```python
from build123d import *

# Parameters (mm, degrees)
F0_W      = 50
F0_H      = 94
F1_DEPTH  = 2.5
F2_W      = 2.5
F2_H      = 10
F3_DEPTH  = 3
F4_R      = 2.5
F5_DEPTH  = 25
F6_W      = 10.5
F6_H      = 16.5188284865
F7_DEPTH  = 8.5
F8_W      = 4
F8_H      = 1
F9_DEPTH  = 3
F11_DEPTH = 82.4821715135
F12_R     = 0.5
F13_R     = 1.25
F14_DEPTH = 2.25
F16_DEPTH = 2
F18_W     = 1.5
F18_H     = 3.5
F19_DEPTH = 3
F20_R     = 1
F21_DEPTH = 6


# Not quite as in the source:
# - a fillet or chamfer that OpenCascade refuses, or shapes differently, is made with other operations: its cross-section is extruded or revolved along the edge and cut away or added


with BuildPart() as f1:
    # F0 (on Right) → F1 (new body)
    with BuildSketch(Plane.YZ):
        with Locations((25, 47)):
            Rectangle(F0_W, F0_H)
    extrude(amount=F1_DEPTH)

    # F2 (on face) → F3 (join)
    with BuildSketch(Plane.XY.offset(94)):
        with Locations((1.25, 40)):
            Rectangle(F2_W, F2_H)
        with Locations((1.25, 10)):
            Rectangle(F2_W, F2_H)
    extrude(amount=F3_DEPTH)

    # F4 (on face) → F5 (cut)
    with BuildSketch(Plane.YZ.offset(2.5)):
        with Locations((25, 40)):
            Circle(F4_R)
        with Locations((25, 54)):
            Circle(F4_R)
    extrude(amount=-F5_DEPTH, mode=Mode.SUBTRACT)

    # F6 (on face) → F7 (join)
    with BuildSketch(Plane.YZ.offset(2.5)):
        with Locations((24.75, 20.2594142432)):
            Rectangle(F6_W, F6_H)
    extrude(amount=F7_DEPTH)

    # F8 (on face) → F9 (join)
    with BuildSketch(Plane.XZ.offset(-19.5)):
        with Locations((6.5, 25.0188284865)):
            Rectangle(F8_W, F8_H)
        with Locations((6.5, 20.0188284865)):
            Rectangle(F8_W, F8_H)
        with Locations((6.5, 15.0188284865)):
            Rectangle(F8_W, F8_H)
    extrude(amount=F9_DEPTH)

    # F10 (on face) → F11 (cut, through all)
    with BuildSketch(Plane(origin=(0, 0, 14.5188284865), x_dir=(1, 0, 0), z_dir=(0, 0, -1))):
        with BuildLine():
            Line((5, -17.5), (5, -19.5))
            Line((5, -19.5), (8, -19.5))
            Line((8, -19.5), (8, -17.5))
            ThreePointArc((8, -17.5), (7.8535533906, -17.1464466094), (7.5, -17))
            Line((7.5, -17), (5.5, -17))
            ThreePointArc((5.5, -17), (5.1464466094, -17.1464466094), (5, -17.5))
        make_face()
    extrude(amount=-F11_DEPTH, mode=Mode.SUBTRACT)

    # F12
    f12_edges = [f1.edges().sort_by_distance(p)[0] for p in [
        (8.5, 16.5, 15.018828),
        (8.5, 16.5, 20.018828),
        (8.5, 16.5, 25.018828),
        (4.5, 16.5, 25.018828),
        (4.5, 16.5, 20.018828),
        (4.5, 16.5, 15.018828),
    ]]
    fillet(f12_edges, radius=F12_R)

    # F13 (on face) → F14 (join)
    with BuildSketch(Plane.YZ.offset(11)):
        with Locations((22.5, 25.5188284865)):
            Circle(F13_R)
        with Locations((22.5, 15)):
            Circle(F13_R)
    extrude(amount=F14_DEPTH)

    # F15 (on face) → F16 (cut)
    with BuildSketch(Plane.YZ.offset(13.25)):
        Polygon((22.2532600164, 25.2959672362), (22.2532600164, 24.5808176696), (22.7513108402, 24.5808176696), (22.7513108402, 25.2959672362), (23.51754345, 25.2959672362), (23.51754345, 25.7301647216), (22.7513108402, 25.7301647216), (22.7513108402, 26.4325458556), (22.2532600164, 26.4325458556), (22.2532600164, 25.7301647216), (21.5636510402, 25.7301647216), (21.5636510402, 25.2959672362), align=None)
        Polygon((22.2596314482, 14.7567068819), (22.2596314482, 14.0415573154), (22.757682272, 14.0415573154), (22.757682272, 14.7567068819), (23.5239148817, 14.7567068819), (23.5239148817, 15.1909043674), (22.757682272, 15.1909043674), (22.757682272, 15.8932855014), (22.2596314482, 15.8932855014), (22.2596314482, 15.1909043674), (21.5700224719, 15.1909043674), (21.5700224719, 14.7567068819), align=None)
    extrude(amount=-F16_DEPTH, mode=Mode.SUBTRACT)

    # F17: fillet of radius 1 on 2 edges, made by hand

    # F17_s1 → F17_t2 (revolve, cut)
    with BuildSketch(Plane.XY.offset(25.5188284865)):
        with BuildLine():
            ThreePointArc((12.25, 23.75), (12.9571067812, 23.4571067812), (13.25, 22.75))
            Line((13.25, 22.75), (13.25, 23.75))
            Line((13.25, 23.75), (12.25, 23.75))
        make_face()
    revolve(axis=Axis((13.25, 22.5, 25.5188284865), (1, 0, 0)), mode=Mode.SUBTRACT)

    # F17_s3 → F17_t4 (revolve, cut)
    with BuildSketch(Plane.XY.offset(15)):
        with BuildLine():
            ThreePointArc((12.25, 23.75), (12.9571067812, 23.4571067812), (13.25, 22.75))
            Line((13.25, 22.75), (13.25, 23.75))
            Line((13.25, 23.75), (12.25, 23.75))
        make_face()
    revolve(axis=Axis((13.25, 22.5, 15), (1, 0, 0)), mode=Mode.SUBTRACT)

    # F18 (on face) → F19 (join)
    with BuildSketch(Plane(origin=(0, 30, 0), x_dir=(-1, 0, 0), z_dir=(0, 1, 0))):
        with Locations((-9.25, 25.5901701748)):
            Rectangle(F18_W, F18_H)
        with Locations((-4.75, 25.6615988507)):
            Rectangle(F18_W, F18_H)
    extrude(amount=F19_DEPTH)

    # F20 (on face) → F21 (cut)
    with BuildSketch(Plane.YZ.offset(10)):
        with Locations((31.5, 25.5901701748)):
            Circle(F20_R)
    extrude(amount=-F21_DEPTH, mode=Mode.SUBTRACT)


solid = f1.part
```
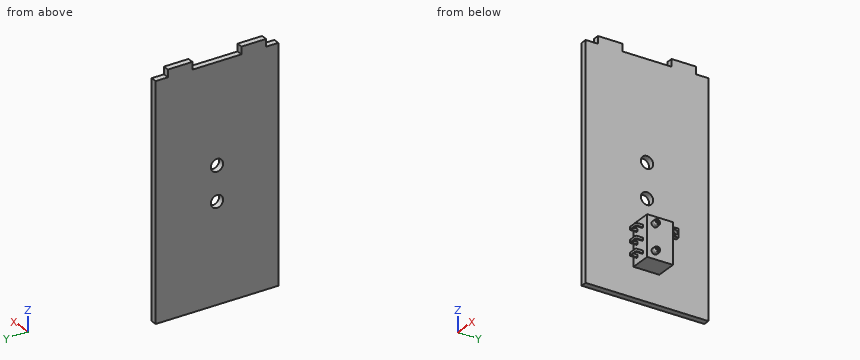
Build history of the part. All positions in model axes, mm. Give positions to 0.01 mm unless a question says otherwise; leave off trailing zeros. Order: outer loops, then holes, each group sorted by start corner. A loop starts at its lowest first (then second) coordinate and runs counter-clockwise, first axis right, second up. Notation, with made-up numbers: M -18.75,88 L -6.75,88 A18 cw -6.75,123 Z; hole C 35,17.25 d2. An arc over 180 degrees is marked long. Write item = value, one per line. Start each with the question number.
(1) Pin check, flat tips, straight feed: pin 1 Ø6 at (x, y) = (9.5, 25.5) entering from -Z; pin 2 Ø0.8 at (x, z) = (6, 15) entering from -Y; pin 3 Ø0.5 at (y, z) = (18, 15) entering from -X; pin 4 Ø0.5 at (y, z) = (18.5, 25) entering from +X. Stop position of each tip, or through.
(2) Slice it at C-C on x = 1.5. Write the cut outline in (y, z), plus the area to 3 significant figures.
(3) Slice it at A-A on y = 31.5. Write the cut outline in (x, z), plus the area to 4 significant figures.
(4) Probe L1, parallel to Z at x = 1.6, y = 25; L2, parallel to Z at x = 9.7, y = 31.5; L3, parallel to Z at x = 4.8, y = 31.5. List the from-to ranges inside material, lowest first. Write a range as [from, to].
(5) Slice it at B-B on z = 54. Write the cut outline in (x, y), plus the area to 4 significant figures.
(6) Slice it at D-D on z = 39. Write the cut outline in (x, y).
Responses:
q1.pin_1 = 12
q1.pin_2 = 16.5
q1.pin_3 = 0
q1.pin_4 = 8.5
q2.outline = M 0,0 L 50,0 L 50,94 L 45,94 L 45,97 L 35,97 L 35,94 L 15,94 L 15,97 L 5,97 L 5,94 L 0,94 Z; hole C 25,40 d5; hole C 25,54 d5
q2.area = 4,720 mm2
q3.outline = M 0,0 L 2.5,0 L 2.5,94 L 0,94 Z; M 4,23.91 L 5.5,23.91 L 5.5,24.59 L 4,24.59 Z; M 4,26.59 L 5.5,26.59 L 5.5,27.41 L 4,27.41 Z; M 8.5,23.84 L 10,23.84 L 10,24.59 L 8.5,24.59 Z; M 8.5,26.59 L 10,26.59 L 10,27.34 L 8.5,27.34 Z
q3.area = 239.5 mm2
q4.L1 = [0, 37.5], [42.5, 51.5], [56.5, 94]
q4.L2 = [23.84, 24.59], [26.59, 27.34]
q4.L3 = [23.91, 24.59], [26.59, 27.41]
q5.outline = M 0,0 L 2.5,0 L 2.5,22.5 L 0,22.5 Z; M 0,27.5 L 2.5,27.5 L 2.5,50 L 0,50 Z
q5.area = 112.5 mm2
q6.outline = M 0,0 L 2.5,0 L 2.5,22.71 L 0,22.71 Z; M 0,27.29 L 2.5,27.29 L 2.5,50 L 0,50 Z
